from build123d import *

# Parameters (mm, degrees)
SKETCH1_W           = 66
SKETCH1_H           = 39
BOSS_EXTRUDE1_DEPTH = 35
SKETCH3_W           = 54
SKETCH3_H           = 39
CUT_EXTRUDE1_DEPTH  = 23
SKETCH4_R           = 11
CUT_EXTRUDE2_DEPTH  = 85.273364713
SKETCH5_R           = 1.5
CUT_EXTRUDE3_DEPTH  = 85.273364713
FILLET2_R           = 0.5


with BuildPart() as part:
    # Sketch1 → Boss-Extrude1 (new body)
    with BuildSketch(Plane(origin=(0, 0, 0), x_dir=(1, 0, 0), z_dir=(0, 1, 0))):
        with Locations((33, 19.5)):
            Rectangle(SKETCH1_W, SKETCH1_H)
    extrude(amount=BOSS_EXTRUDE1_DEPTH)

    # Sketch3 → Cut-Extrude1 (cut)
    with BuildSketch(Plane(origin=(0, 35, 0), x_dir=(1, 0, 0), z_dir=(0, 1, 0))):
        with Locations((33, 19.5)):
            Rectangle(SKETCH3_W, SKETCH3_H)
    extrude(amount=-CUT_EXTRUDE1_DEPTH, mode=Mode.SUBTRACT)

    # Sketch4 → Cut-Extrude2 (cut, through all)
    with BuildSketch(Plane(origin=(66, 0, 0), x_dir=(0, 0, -1), z_dir=(1, 0, 0))):
        with Locations((19.5, 0)):
            Circle(SKETCH4_R)
    extrude(amount=-CUT_EXTRUDE2_DEPTH, mode=Mode.SUBTRACT)

    # Sketch5 → Cut-Extrude3 (cut, through all)
    with BuildSketch(Plane(origin=(0, 35, 0), x_dir=(1, 0, 0), z_dir=(0, 1, 0))):
        with Locations(Location((3, 3, 0), (0, 0, 270))):
            Circle(SKETCH5_R)
        with Locations(Location((63, 3, 0), (0, 0, 270))):
            Circle(SKETCH5_R)
        with Locations(Location((63, 36, 0), (0, 0, 270))):
            Circle(SKETCH5_R)
        with Locations(Location((3, 36, 0), (0, 0, 270))):
            Circle(SKETCH5_R)
    extrude(amount=-CUT_EXTRUDE3_DEPTH, mode=Mode.SUBTRACT)

    # Fillet2
    fillet2_edges = [part.edges().sort_by_distance(p)[0] for p in [
        (60, 23.5, 0),
        (60, 23.5, -39),
        (6, 23.5, -39),
        (6, 23.5, 0),
        (0, 17.5, -39),
        (66, 17.5, -39),
        (66, 17.5, 0),
        (0, 17.5, 0),
    ]]
    fillet(fillet2_edges, radius=FILLET2_R)


solid = part.part
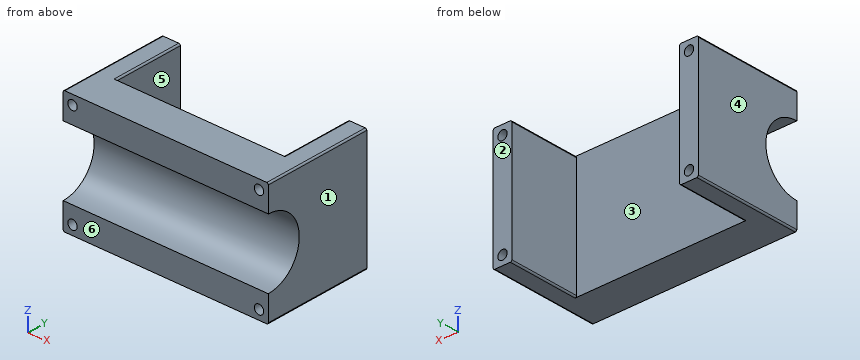
The listing builds one solid part. Answer for the finished solid, in the listing's coordinates (mm). Face numbers are marked on the shaded views. A direction names the side the tool comes from. Give positions to 0.01 mm unless a question says otherwise; leave off trailing zeros. Write each loop counter-clockwise with the first axis right and the second up, starting at its lowest first coordinate (ties: lowest second). Pieces come first, ordered by that corner, then holes. Notation, with made-up numbers: (88.25, 12) -> (96.25, 12) arc R11 ccw to (96.25, 25) -> close; hole circle Ø4 at (54.25, 2.5). An arc over 180 degrees is marked (long way). One line per question, with ' | ' between items. Start each with the question number.
1. Find the intervals of material crossed by probe 1 along X at (y, z) = (20.5, -36); probe 2 along X at (y, z) = (7, -36); probe 3 along X at (y, z) = (17.5, -12.5), in increasing order.
2. Section C-C (z = -36) is taken. Determine the outline of the cut face in (x, y).
3. Section A-A (y = 24.5) is taken. Determine the outline of the cut face in (x, z), plus the area to 3 significant figures.
4. For a pull along X with two mould halves and no side action, classify the marked faces 1, 2, 3 and 4 as pulls with the +X half, pulls with the -X half, needs draft (parallel to the pull), parting line crosses it, or undercut.
5. For the marked faces 5 and 6, determine the directions among +Z, -Z, +X, -X, +Y, -Y from which every point of the face is accessible in a straight line to the end or side of a thin tool.
6. Section D-D (z = -19.5) is taken. Determine the outline of the cut face in (x, y).
7. Given pin 1 Ø4 at (x, z) = (19, -7.5) entering from +Y; pin 2 Ø12 at (x, y) = (7, 28.5) entering from -Z, each flat-ended and moving along its own axis, determine where each tip first touches the part or whether it passes through.
8. Section B-B (x = 3) is taken. Determine the outline of the cut face in (y, z), plus the area to 3 significant figures.
Response values:
1) probe 1: 0 to 1.5, 4.5 to 6, 60 to 61.5, 64.5 to 66 | probe 2: 0 to 1.5, 4.5 to 61.5, 64.5 to 66 | probe 3: 0 to 6, 60 to 66
2) outline: (0, 0) -> (1.5, 0) -> (1.5, 35) -> (0, 35) -> close; (4.5, 0) -> (61.5, 0) -> (61.5, 35) -> (60, 35) -> (60, 12) -> (6, 12) -> (6, 35) -> (4.5, 35) -> close; (64.5, 0) -> (66, 0) -> (66, 35) -> (64.5, 35) -> close
3) outline: (0, -38.5) arc R0.5 ccw to (0.5, -39) -> (5.5, -39) arc R0.5 ccw to (6, -38.5) -> (6, -0.5) arc R0.5 ccw to (5.5, 0) -> (0.5, 0) arc R0.5 ccw to (0, -0.5) -> close; (60, -38.5) arc R0.5 ccw to (60.5, -39) -> (65.5, -39) arc R0.5 ccw to (66, -38.5) -> (66, -0.5) arc R0.5 ccw to (65.5, 0) -> (60.5, 0) arc R0.5 ccw to (60, -0.5) -> close; hole circle Ø3 at (3, -36); hole circle Ø3 at (3, -3); hole circle Ø3 at (63, -36); hole circle Ø3 at (63, -3) | area: 439 mm2
4) face 1: pulls with the +X half | face 2: needs draft | face 3: undercut | face 4: pulls with the -X half
5) face 5: +Z, -Z, +Y | face 6: +Z, -Z, +X, -X, -Y
6) outline: (0, 11) -> (66, 11) -> (66, 35) -> (60, 35) -> (60, 12) -> (6, 12) -> (6, 35) -> (0, 35) -> close
7) pin 1: y = 12 | pin 2: z = -39
8) outline: (0, -39) -> (35, -39) -> (35, -37.5) -> (0, -37.5) -> close; (0, -34.5) -> (35, -34.5) -> (35, -4.5) -> (0, -4.5) -> (0, -8.5) arc R11 cw to (0, -30.5) -> close; (0, -1.5) -> (35, -1.5) -> (35, 0) -> (0, 0) -> close | area: 965 mm2
